CAD build for the part. Positions are in the model's coordinates, mm. Face numbers are marked on the shaded views. A direction names the side the tool comes from. Round coordinates to 2 decimals unless told otherwise and drop trailing zeros.
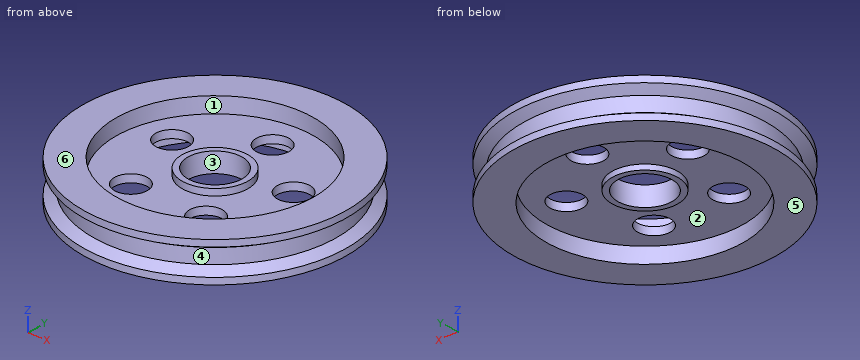
```python
from build123d import *

# Parameters (mm, degrees)
SKETCH1_R                = 20
SKETCH1_R_2              = 4
BOSS_EXTRUDE1_DEPTH      = 3
SKETCH3_R                = 15
CUT_EXTRUDE1_DEPTH       = 2.4
SKETCH4_R                = 2.5
CUT_EXTRUDE2_DEPTH       = 4.6
CIRPATTERN1_COUNT        = 5
SKETCH14_R               = 5
BOSS_EXTRUDE3_DEPTH      = 1
BOSS_EXTRUDE3_DEPTH_BACK = 2
SKETCH16_R               = 4.125
CUT_EXTRUDE3_DEPTH       = 5.6


with BuildPart() as part:
    # Sketch1 → Boss-Extrude1 (new body, symmetric)
    with BuildSketch(Plane.XY):
        Circle(SKETCH1_R)
        Circle(SKETCH1_R_2, mode=Mode.SUBTRACT)
    extrude(amount=BOSS_EXTRUDE1_DEPTH, both=True)

    # Sketch3 → Cut-Extrude1 (cut)
    with BuildSketch(Plane.XY.offset(3)):
        Circle(SKETCH3_R)
    cut_extrude1 = extrude(amount=-CUT_EXTRUDE1_DEPTH, mode=Mode.SUBTRACT)

    # Mirror1: Cut-Extrude1 across plane
    add(cut_extrude1.mirror(Plane.XY), mode=Mode.SUBTRACT)

    # Sketch4 → Cut-Extrude2 (cut, through all)
    with BuildSketch(Plane.XY.offset(0.6)):
        with Locations((0, 10)):
            Circle(SKETCH4_R)
    cut_extrude2 = extrude(amount=-CUT_EXTRUDE2_DEPTH, mode=Mode.SUBTRACT)

    # CirPattern1: Cut-Extrude2 ×5 about axis
    cirpattern1_axis = Axis((0, 0, 0), (0, 0, 1))
    for i in range(1, CIRPATTERN1_COUNT):
        add(cut_extrude2.rotate(cirpattern1_axis, i * 360 / CIRPATTERN1_COUNT), mode=Mode.SUBTRACT)

    # Sketch5 → Cut-Revolve1 (revolve, cut)
    with BuildSketch(Plane(origin=(0, 0, 0), x_dir=(1, 0, 0), z_dir=(0, 1, 0))):
        Polygon((20, 2), (18.5, 1.133974596), (18.5, -1.133974596), (20, -2), align=None)
    revolve(axis=Axis((0, 0, 0), (0, 0, -1)), mode=Mode.SUBTRACT)

    # Sketch14 → Boss-Extrude3 (add, two sides)
    with BuildSketch(Plane.XY.offset(0.6)) as boss_extrude3_sk:
        Circle(SKETCH14_R)
    extrude(amount=BOSS_EXTRUDE3_DEPTH)
    extrude(boss_extrude3_sk.sketch, amount=-BOSS_EXTRUDE3_DEPTH_BACK)

    # Sketch16 → Cut-Extrude3 (cut, through all)
    with BuildSketch(Plane.XY.offset(1.6)):
        Circle(SKETCH16_R)
    extrude(amount=-CUT_EXTRUDE3_DEPTH, mode=Mode.SUBTRACT)


solid = part.part
```
Item 1: 3-axis set-ups, long thin cutter, end or side, ignore diameter. For the marked faces 1, 2 and 3: which of +Z, -Z, +X, -X, +Y, -Y reach the whole face in a straight line?
Answers follow:
face 1: +Z
face 2: -Z
face 3: +Z, -Z
Item 2: Probe line 1 (Y direction, x = -3, z = -0.8); line 2 (Y direction, x = 0, z = 0.4) (3 decimals); line 3 (Y direction, x = 0, z = 2.45). List the from-to ranges inside material, lowest first.
Answers follow:
line 1: y = -18.26 to -14.7, -4 to -2.83, 2.83 to 4, 14.7 to 18.26
line 2: y = -18.5 to -4.125, 4.125 to 7.5, 12.5 to 18.5
line 3: y = -20 to -15, 15 to 20
Item 3: Two-plate mould, pull along Z, no slides. Class the marked faces 4, 5 and 6: released by +Z, released by -Z, zero draft, split by the parting line, or undercut.
Answers follow:
face 4: undercut
face 5: released by -Z
face 6: released by +Z
Item 4: Cut at B-B, the plane x = 0. State how many separate pieces and enclosed holes the cut face has, plus the area to 3 significant figures.
Answers follow:
separate pieces: 3
enclosed holes: 0
area: 73.8 mm2
Item 5: Flat gauge pins, fed straight in: P1, Ø18, axis at x = 0, y = 0, coming from the +Z side; P2, Ø4, axis at x = 9.51, y = 3.09, coming from the -Z side; P3, Ø3, axis at x = 1.5, y = 2.5, coming from the -Z side; P4, Ø1, axis at x = 6, z = -2, coming from the +Y side. Where does each tip first touch, or does it go through?
Answers follow:
P1: stops at z = 1.6
P2: passes through
P3: stops at z = -1.4
P4: stops at y = 19.23
